Input: part model. Units: mm. Frame: model coordinates. Give positions to 0.01 mm unless a question says otherwise; leave off trailing zeros. Loops run counter-clockwise (first coordinate to the right, second up) from the corner with the lowest first, then second, coordinate; pieces in that order, holes last. Notation, with made-up numbers: M 30,-17.5 L 48,-17.5 A37 cw 48,20.5 Z; hole C 68.5,38.25 d6. An arc over 180 degrees is marked long. Use CSV: the item, a comma, the result in double quotes. Start each with the question number.
from build123d import *

# Parameters (mm, degrees)
ESQUISSE1_W        = 40
ESQUISSE1_H        = 80
ESQUISSE1_R        = 2.75
BOSS_EXTRU_1_DEPTH = 5


with BuildPart() as part:
    # Esquisse1 → Boss.-Extru.1 (new body)
    with BuildSketch(Plane.XY):
        with Locations((-40.349893162, -20.555555556)):
            Rectangle(ESQUISSE1_W, ESQUISSE1_H)
        with Locations((-50.349893162, 9.444444444)):
            Circle(ESQUISSE1_R, mode=Mode.SUBTRACT)
        with Locations((-30.349893162, 9.444444444)):
            Circle(ESQUISSE1_R, mode=Mode.SUBTRACT)
        with Locations((-30.349893162, -10.555555556)):
            Circle(ESQUISSE1_R, mode=Mode.SUBTRACT)
        with Locations((-30.349893162, -30.555555556)):
            Circle(ESQUISSE1_R, mode=Mode.SUBTRACT)
        with Locations((-30.349893162, -50.555555556)):
            Circle(ESQUISSE1_R, mode=Mode.SUBTRACT)
        with Locations((-50.349893162, -10.555555556)):
            Circle(ESQUISSE1_R, mode=Mode.SUBTRACT)
        with Locations((-50.349893162, -30.555555556)):
            Circle(ESQUISSE1_R, mode=Mode.SUBTRACT)
        with Locations((-50.349893162, -50.555555556)):
            Circle(ESQUISSE1_R, mode=Mode.SUBTRACT)
    extrude(amount=BOSS_EXTRU_1_DEPTH)


solid = part.part
Item 1: Section D-D (x = -52). Output: boundary loops of the cut face in (y, z), then the cut area to 3 significant figures.
Item 2: First-contact query: pin 1 Ø5 at (x, y) = (-30.35, 9.44) entering from -Z. Flat tip, straight axial feed; report the tip coordinate or a pass-through.
Item 3: Section A-A (x = -31). Output: boundary loops of the cut face in (y, z).
Item 4: Section B-B (z = 4.25). State how many separate pieces and enclosed holes the cut face has, then the cut area to 3 significant figures.
Item 5: Mould query, pull axis X, two halves, no side actions, for faces 1 (the cylindrical face through (-47.727, -49.73, 2.465)), 2 (the flat face through (-41, -20, 5)), 3 (the flat face through (-60.35, -21, 2)). Classes: +X half, -X half, draft (parallel to the pull), parting line (faces both ways), or undercut.
Item 6: Material intervals for line 1 (X direction, y = -51.5, z = 4.45); line 2 (Y direction, x = -48, z = 4); line 3 (Y direction, x = -30, z = 4.1), sorted ascending.
Item 7: Section C-C (y = 8.5). Output: boundary loops of the cut face in (x, z), then the cut area to 3 significant figures.
Recorded:
1,outline,"M -60.56,0 L -52.76,0 L -52.76,5 L -60.56,5 Z; M -48.36,0 L -32.76,0 L -32.76,5 L -48.36,5 Z; M -28.36,0 L -12.76,0 L -12.76,5 L -28.36,5 Z; M -8.36,0 L 7.24,0 L 7.24,5 L -8.36,5 Z; M 11.64,0 L 19.44,0 L 19.44,5 L 11.64,5 Z"
1,area,"312 mm²"
2,pin 1,"through"
3,outline,"M -60.56,0 L -53.23,0 L -53.23,5 L -60.56,5 Z; M -47.88,0 L -33.23,0 L -33.23,5 L -47.88,5 Z; M -27.88,0 L -13.23,0 L -13.23,5 L -27.88,5 Z; M -7.88,0 L 6.77,0 L 6.77,5 L -7.88,5 Z; M 12.12,0 L 19.44,0 L 19.44,5 L 12.12,5 Z"
4,separate pieces,"1"
4,enclosed holes,"8"
4,area,"3,010 mm²"
5,face 1,"undercut"
5,face 2,"draft"
5,face 3,"-X half"
6,line 1,"-60.35 to -52.93, -47.77 to -32.93, -27.77 to -20.35"
6,line 2,"-60.56 to -51.98, -49.13 to -31.98, -29.13 to -11.98, -9.13 to 8.02, 10.87 to 19.44"
6,line 3,"-60.56 to -53.28, -47.83 to -33.28, -27.83 to -13.28, -7.83 to 6.72, 12.17 to 19.44"
7,outline,"M -60.35,0 L -52.93,0 L -52.93,5 L -60.35,5 Z; M -47.77,0 L -32.93,0 L -32.93,5 L -47.77,5 Z; M -27.77,0 L -20.35,0 L -20.35,5 L -27.77,5 Z"
7,area,"148 mm²"
